from build123d import *

# Parameters (mm, degrees)
SKETCH1_W           = 48
SKETCH1_H           = 270
SKETCH1_W_2         = 7.1
SKETCH1_H_2         = 264
BOSS_EXTRUDE1_DEPTH = 1
FILLET1_R           = 3


with BuildPart() as part:
    # Sketch1 → Boss-Extrude1 (new body)
    with BuildSketch(Plane(origin=(0, 0, 0), x_dir=(1, 0, 0), z_dir=(0, 1, 0))):
        Rectangle(SKETCH1_W, SKETCH1_H)
        with Locations((-16.45, 0)):
            Rectangle(SKETCH1_W_2, SKETCH1_H_2, mode=Mode.SUBTRACT)
        with Locations((16.45, 0)):
            Rectangle(SKETCH1_W_2, SKETCH1_H_2, mode=Mode.SUBTRACT)
    extrude(amount=BOSS_EXTRUDE1_DEPTH)

    # Fillet1
    fillet1_edges = [part.edges().sort_by_distance(p)[0] for p in [
        (-20, 0.5, -132),
        (-20, 0.5, 132),
        (-12.9, 0.5, 132),
        (-12.9, 0.5, -132),
        (20, 0.5, 132),
        (20, 0.5, -132),
        (12.9, 0.5, -132),
        (12.9, 0.5, 132),
    ]]
    fillet(fillet1_edges, radius=FILLET1_R)


solid = part.part
For this review, take the finished solid that the model builds, in its own axes (mm). Coordinates: 2 decimals unless noted, no trailing zeros. Loops run counter-clockwise (first coordinate to the right, second up) from the corner with the lowest first, then second, coordinate; pieces in that order, holes last. Notation, with made-up numbers: (-30, -34) - (-4, -34) arc R27 ccw to (-4, -2) - close; hole circle Ø11 at (75.5, 70.25). An arc over 180 degrees is marked (long way). Return JSON: item names as keys, results as strings.
Item 1: For line 1 (X direction, y = 0.2, z = 80.5); line 2 (Z direction, x = -15.5, y = 0.1); line 3 (Z direction, x = -18, y = 0.1), list the stretches that pass through material, from the lowest coordinate up.
Determined:
{"line 1": "x = -24 to -20, -12.9 to 12.9, 20 to 24", "line 2": "z = -135 to -131.97, 131.97 to 135", "line 3": "z = -135 to -131.83, 131.83 to 135"}
Item 2: Take a section at A-A (z = -91.5). Give the boundary of the cut face in (x, y), then the cut area to 3 significant figures.
Determined:
{"outline": "(-24, 0) - (-20, 0) - (-20, 1) - (-24, 1) - close; (-12.9, 0) - (12.9, 0) - (12.9, 1) - (-12.9, 1) - close; (20, 0) - (24, 0) - (24, 1) - (20, 1) - close", "area": "33.8 mm2"}
Item 3: Take a section at B-B (y = 0.3). Give the boundary of the cut face in (x, z), then the cut area to 3 significant figures.
Determined:
{"outline": "(-24, -135) - (24, -135) - (24, 135) - (-24, 135) - close; hole (-20, -129) arc R3 ccw to (-17, -132) - (-15.9, -132) arc R3 ccw to (-12.9, -129) - (-12.9, 129) arc R3 ccw to (-15.9, 132) - (-17, 132) arc R3 ccw to (-20, 129) - close; hole (12.9, -129) arc R3 ccw to (15.9, -132) - (17, -132) arc R3 ccw to (20, -129) - (20, 129) arc R3 ccw to (17, 132) - (15.9, 132) arc R3 ccw to (12.9, 129) - close", "area": "9,230 mm2"}
